The listing builds one solid part. Answer for the finished solid, in the listing's coordinates (mm). Face numbers are marked on the shaded views. Coordinates: 2 decimals unless noted, no trailing zeros. Write each loop counter-clockwise with the first axis right and the second up, starting at its lowest first coordinate (ties: lowest second). Pieces come first, ordered by that corner, then holes.
from build123d import *

# Parameters (mm, degrees)
SKETCH1_R             = 20
SKETCH1_R_2           = 37.5
SKETCH1_R_3           = 15
SKETCH1_R_4           = 32.5
SKETCH1_R_5           = 23.5
BOSS_EXTRUDE1_DEPTH   = 12
SKETCH2_R             = 2
CUT_EXTRUDE1_DEPTH    = 13
CIRPATTERN1_COUNT     = 8
SKETCH3_R             = 2
CUT_EXTRUDE2_DEPTH    = 13
CIRPATTERN2_COUNT     = 6
SKETCH6_R             = 2
CUT_EXTRUDE4_DEPTH    = 235.906743238
F_1_0MM_DOWEL_HOLE1_D = 3.3
LPATTERN1_COUNT       = 5
LPATTERN1_PITCH       = 56.5
MIRROR1_COPY_1_D      = 3.3
MIRROR1_COPY_2_D      = 3.3
MIRROR1_COPY_3_D      = 3.3
MIRROR1_COPY_4_D      = 3.3
SKETCH10_W            = 9
SKETCH10_H            = 65
BOSS_EXTRUDE2_DEPTH   = 12
FILLET1_R             = 5
SKETCH12_R            = 2.5
CUT_EXTRUDE5_DEPTH    = 12
FILLET1_OF_MIRROR2_R  = 5


with BuildPart() as part:
    # Sketch1 → Boss-Extrude1 (new body)
    # profile 1 of 3: a face of its own
    with BuildSketch(Plane.XY):
        with BuildLine():
            ThreePointArc((32.5, 199.083522771), (0, 166.583522771), (-32.5, 199.083522771))
            Line((-32.5, 199.083522771), (-32.5, -89.208190296))
            ThreePointArc((-32.5, -89.208190296), (0, -70.416477229), (32.5, -89.208190296))
            Line((32.5, -89.208190296), (32.5, 199.083522771))
        make_face()
        with Locations((0, -27.916477229)):
            Circle(SKETCH1_R, mode=Mode.SUBTRACT)
    # profile 2 of 3: a face of its own
    with BuildSketch(Plane.XY):
        with Locations((0, -107.916477229)):
            Circle(SKETCH1_R_2)
        with Locations((0, -107.916477229)):
            Circle(SKETCH1_R_3, mode=Mode.SUBTRACT)
    # profile 3 of 3: a face of its own
    with BuildSketch(Plane.XY):
        with Locations((0, 199.083522771)):
            Circle(SKETCH1_R_4)
        with Locations((0, 199.083522771)):
            Circle(SKETCH1_R_5, mode=Mode.SUBTRACT)
    extrude(amount=BOSS_EXTRUDE1_DEPTH)

    # Sketch2 → Cut-Extrude1 (cut)
    with BuildSketch(Plane(origin=(0, 0, 0), x_dir=(-1, 0, 0), z_dir=(0, 0, -1))):
        with Locations((-20.7, -107.916477229)):
            Circle(SKETCH2_R)
    cut_extrude1 = extrude(amount=-CUT_EXTRUDE1_DEPTH, mode=Mode.SUBTRACT)

    # CirPattern1: Cut-Extrude1 ×8 about axis
    cirpattern1_axis = Axis((0, -107.916477229, 0), (0, 0, 1))
    for i in range(1, CIRPATTERN1_COUNT):
        add(cut_extrude1.rotate(cirpattern1_axis, i * 360 / CIRPATTERN1_COUNT), mode=Mode.SUBTRACT)

    # Sketch3 → Cut-Extrude2 (cut)
    with BuildSketch(Plane(origin=(0, 0, 0), x_dir=(-1, 0, 0), z_dir=(0, 0, -1))):
        with Locations((0, 225.783522771)):
            Circle(SKETCH3_R)
    cut_extrude2 = extrude(amount=-CUT_EXTRUDE2_DEPTH, mode=Mode.SUBTRACT)

    # CirPattern2: Cut-Extrude2 ×6 about axis
    cirpattern2_axis = Axis((0, 199.083522771, 0), (0, 0, 1))
    for i in range(1, CIRPATTERN2_COUNT):
        add(cut_extrude2.rotate(cirpattern2_axis, i * 360 / CIRPATTERN2_COUNT), mode=Mode.SUBTRACT)

    # Sketch6 → Cut-Extrude4 (cut, through all)
    with BuildSketch(Plane(origin=(0, 0, 0), x_dir=(-1, 0, 0), z_dir=(0, 0, -1))):
        with Locations((-5, 227.083522771)):
            Circle(SKETCH6_R)
        with Locations((5, 227.083522771)):
            Circle(SKETCH6_R)
    extrude(amount=-CUT_EXTRUDE4_DEPTH, mode=Mode.SUBTRACT)

    # Ø1.0mm Dowel Hole1 (through all)
    with Locations(Plane(origin=(0, 0, 0), x_dir=(-1, 0, 0), z_dir=(0, 0, -1))):
        with Locations((-28.5, 199.083522771)):
            f_1_0mm_dowel_hole1 = Hole(F_1_0MM_DOWEL_HOLE1_D / 2)

    # LPattern1: Ø1.0mm Dowel Hole1 ×5
    with Locations(*[(0, -i * LPATTERN1_PITCH, 0) for i in range(1, LPATTERN1_COUNT)]):
        add(f_1_0mm_dowel_hole1, mode=Mode.SUBTRACT)

    # Mirror1: Ø1.0mm Dowel Hole1 across plane
    add(f_1_0mm_dowel_hole1.mirror(Plane(origin=(0, 0, 0), x_dir=(0, 0, 1), z_dir=(1, 0, 0))), mode=Mode.SUBTRACT)

    # Mirror1 copy 1 (through all)
    with Locations(Plane(origin=(0, -56.5, 0), x_dir=(1, 0, 0), z_dir=(0, 0, -1))):
        with Locations((-28.5, -199.083522771)):
            Hole(MIRROR1_COPY_1_D / 2)

    # Mirror1 copy 2 (through all)
    with Locations(Plane(origin=(0, -113, 0), x_dir=(1, 0, 0), z_dir=(0, 0, -1))):
        with Locations((-28.5, -199.083522771)):
            Hole(MIRROR1_COPY_2_D / 2)

    # Mirror1 copy 3 (through all)
    with Locations(Plane(origin=(0, -169.5, 0), x_dir=(1, 0, 0), z_dir=(0, 0, -1))):
        with Locations((-28.5, -199.083522771)):
            Hole(MIRROR1_COPY_3_D / 2)

    # Mirror1 copy 4 (through all)
    with Locations(Plane(origin=(0, -226, 0), x_dir=(1, 0, 0), z_dir=(0, 0, -1))):
        with Locations((-28.5, -199.083522771)):
            Hole(MIRROR1_COPY_4_D / 2)

    # Sketch10 → Boss-Extrude2 (add)
    with BuildSketch(Plane.XY.offset(12)):
        with Locations((-37, -27.916477229)):
            Rectangle(SKETCH10_W, SKETCH10_H)
    boss_extrude2 = extrude(amount=-BOSS_EXTRUDE2_DEPTH)

    # Fillet1
    fillet1_edges = [part.edges().sort_by_distance(p)[0] for p in [
        (-41.5, -60.416477229, 6),
        (-41.5, 4.583522771, 6),
    ]]
    fillet(fillet1_edges, radius=FILLET1_R)

    # Sketch12 → Cut-Extrude5 (cut)
    with BuildSketch(Plane.XY.offset(12)):
        with Locations((-33, -16.416477229)):
            Circle(SKETCH12_R)
        with Locations((-33, -39.416477229)):
            Circle(SKETCH12_R)
    cut_extrude5 = extrude(amount=-CUT_EXTRUDE5_DEPTH, mode=Mode.SUBTRACT)

    # Mirror2: Boss-Extrude2, Cut-Extrude5 across plane
    add(boss_extrude2.mirror(Plane(origin=(0, 0, 0), x_dir=(0, 0, 1), z_dir=(1, 0, 0))))
    add(cut_extrude5.mirror(Plane(origin=(0, 0, 0), x_dir=(0, 0, 1), z_dir=(1, 0, 0))), mode=Mode.SUBTRACT)

    # Fillet1 of Mirror2
    fillet1_of_mirror2_edges = [part.edges().sort_by_distance(p)[0] for p in [
        (41.5, -60.416477229, 6),
        (41.5, 4.583522771, 6),
    ]]
    fillet(fillet1_of_mirror2_edges, radius=FILLET1_OF_MIRROR2_R)


solid = part.part
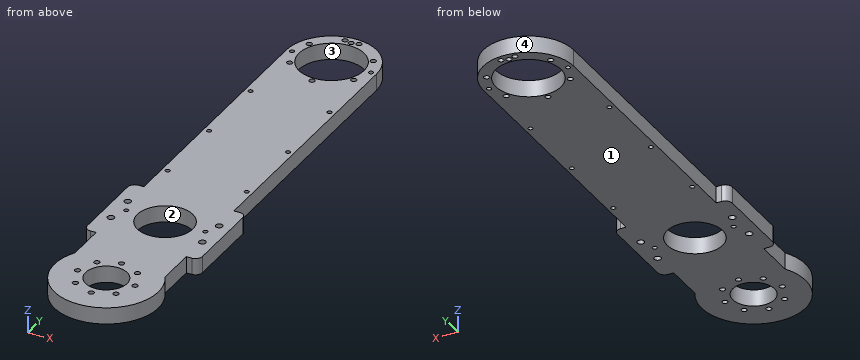
Q1. The part is cut by section C-C, the plane z = 9.25. State how many separate pieces and enclosed holes the cut face has, then the cut area to 3 significant figures.
Answers below:
separate pieces: 1
enclosed holes: 33
area: 21,000 mm2
Q2. Determine the mould class of the marked faces 1, 2, 3 and 4 for opening direction X: released by +X, released by -X, zero draft, split by the parting line, or undercut.
Answers below:
face 1: zero draft
face 2: undercut
face 3: undercut
face 4: split by the parting line
Q3. The part is cut by section A-A, the plane y = -32. Write down the section's boundary in (x, z).
Answers below:
outline: (-41.5, 0) - (-19.58, 0) - (-19.58, 12) - (-41.5, 12) - close; (19.58, 0) - (41.5, 0) - (41.5, 12) - (19.58, 12) - close
Q4. Find the intervals of material crossed by probe 1 along Y at (x, z) = (-28.5, 4); probe 2 along Y at (x, z) = (20.5, 1.5); probe 3 along Y at (x, z) = (-5, 6.5), in increasing order.
Answers below:
probe 1: y = -132.29 to -28.57, -25.27 to 27.93, 31.23 to 84.43, 87.73 to 140.93, 144.23 to 197.43, 200.73 to 214.7
probe 2: y = -139.32 to -109.91, -105.93 to 187.59, 210.57 to 224.3
probe 3: y = -145.08 to -122.06, -93.77 to -47.28, -8.55 to 176.12, 222.05 to 225.08, 229.08 to 231.2
Q5. Given pin 1 (4 mm diameter, centred on y = 89.5, z = 5, fed in from -X); pin 2 (1 mm diameter, centred on y = 193, z = 8, fed in from +X); pin 3 (3 mm diameter, centred on y = -89.5, z = 5.5, fed in from -X), each flat-ended and moving along its own axis, determine where each tip first touches the part or whether it passes through.
Answers below:
pin 1: stops at x = -32.5
pin 2: stops at x = 32.5
pin 3: stops at x = -33.47
Q6. The part is cut by section B-B, the plane y = 106.5. Write down the section's boundary in (x, z), then the cut area to 3 significant figures.
Answers below:
outline: (-32.5, 0) - (32.5, 0) - (32.5, 12) - (-32.5, 12) - close
area: 780 mm2
